Check sheet for the drawn part. Datum: minimum x, y, z corner. Units: mm. A direction names the side the tool comes from. Coordinates: 2 decimals unless noted, no trailing zeros. Write each loop counter-clockwise with the first axis right and the second up, starting at its lowest first coordinate (ties: lowest second). Pieces come first, ordered by that corner, then holes. Notation, with made-up numbers: (-16, 3.25) -> (39, 3.25) arc R17 cw to (39, 7.25) -> close; hole circle Ø8 at (-35, 9). An arc over 180 degrees is marked (long way). Write item = value, one per line. Start each with the question number.
(1) Section check C-C (y = 23.5). Record the cut outline in (x, z).
(2) Gauge pin test, flat ends, axial feed: pin 1 Ø3 at (y, z) = (16.5, 13) entering from -X; pin 2 Ø7 at (x, z) = (29, 16.5) entering from +Y; pin 3 Ø7.5 at (x, y) = (24.5, 17.5) entering from +Z. Record the tip position at first contact, or that the pin passes through.
(3) Section check A-A (x = 12.7). Record the cut outline in (y, z), plus the area to 3 significant figures.
(4) Section check B-B (z = 19.75). Record the cut outline in (x, y) (1 decimal).
(5) Mould release check, pull along X, two halves, no side actions. Record for the marked faces 1, 2, 3 and 4: released by +X, released by -X, zero draft, split by the parting line, or undercut.
(6) Material ranges on probe 1 along X at (y, z) = (4.75, 19.05) (1 decimal); probe 2 along Y at (x, z) = (38.1, 7.5); probe 3 along Y at (x, z) = (12.7, 3.25), recorded low to high. Write a range as [from, to].
(7) Set-up check for the marked faces 5 and 6: record each of +Z, -Z, +X, -X, +Y, -Y from which the full face is reachable in a straight line by a thin tool's end or side.
(8) Section check D-D (y = 20.25). Record the cut outline in (x, z).
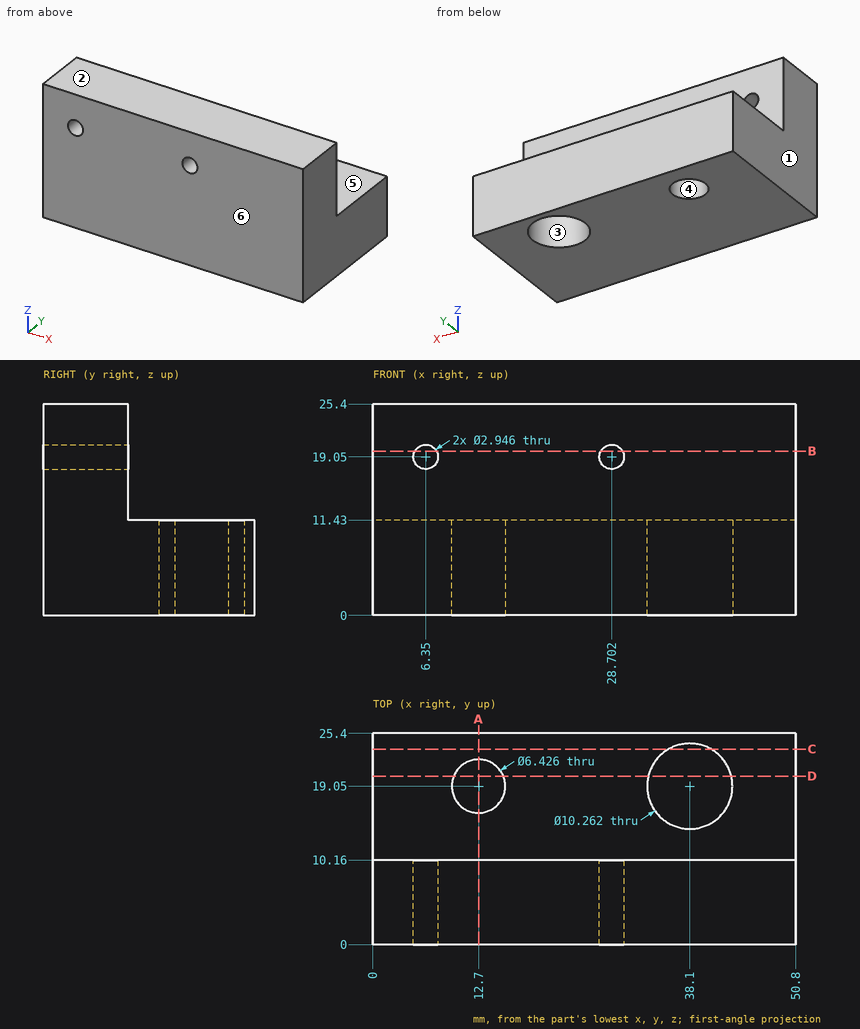
Response:
q1.outline = (0, 0) -> (35.55, 0) -> (35.55, 11.43) -> (0, 11.43) -> close; (40.65, 0) -> (50.8, 0) -> (50.8, 11.43) -> (40.65, 11.43) -> close
q2.pin_1 = through
q2.pin_2 = 10.16
q2.pin_3 = 11.43
q3.outline = (0, 0) -> (15.84, 0) -> (15.84, 11.43) -> (10.16, 11.43) -> (10.16, 25.4) -> (0, 25.4) -> close; (22.26, 0) -> (25.4, 0) -> (25.4, 11.43) -> (22.26, 11.43) -> close
q3.area = 359 mm2
q4.outline = (0, 0) -> (5.1, 0) -> (5.1, 10.2) -> (0, 10.2) -> close; (7.6, 0) -> (27.4, 0) -> (27.4, 10.2) -> (7.6, 10.2) -> close; (30, 0) -> (50.8, 0) -> (50.8, 10.2) -> (30, 10.2) -> close
q5.face_1 = released by -X
q5.face_2 = zero draft
q5.face_3 = undercut
q5.face_4 = undercut
q6.probe_1 = [0, 4.9], [7.8, 27.2], [30.2, 50.8]
q6.probe_2 = [0, 13.92], [24.18, 25.4]
q6.probe_3 = [0, 15.84], [22.26, 25.4]
q7.face_5 = +Z, +X, -X, +Y
q7.face_6 = +Z, -Z, +X, -X, -Y
q8.outline = (0, 0) -> (9.72, 0) -> (9.72, 11.43) -> (0, 11.43) -> close; (15.68, 0) -> (33.11, 0) -> (33.11, 11.43) -> (15.68, 11.43) -> close; (43.09, 0) -> (50.8, 0) -> (50.8, 11.43) -> (43.09, 11.43) -> close
